```python
from build123d import *

# Parameters (mm, degrees)
SKETCH1_R           = 22.5
BOSS_EXTRUDE1_DEPTH = 20
SKETCH2_R           = 30
BOSS_EXTRUDE2_DEPTH = 40
SKETCH3_R           = 25
BOSS_EXTRUDE3_DEPTH = 30
SKETCH4_R           = 20
BOSS_EXTRUDE4_DEPTH = 25
SKETCH5_R           = 15
CUT_EXTRUDE1_DEPTH  = 116


with BuildPart() as part:
    # Sketch1 → Boss-Extrude1 (new body)
    with BuildSketch(Plane(origin=(0, 0, 0), x_dir=(0, 0, -1), z_dir=(1, 0, 0))):
        Circle(SKETCH1_R)
    extrude(amount=BOSS_EXTRUDE1_DEPTH)

    # Sketch2 → Boss-Extrude2 (add)
    with BuildSketch(Plane(origin=(20, 0, 0), x_dir=(0, 0, -1), z_dir=(1, 0, 0))):
        Circle(SKETCH2_R)
    extrude(amount=BOSS_EXTRUDE2_DEPTH)

    # Sketch3 → Boss-Extrude3 (add)
    with BuildSketch(Plane(origin=(60, 0, 0), x_dir=(0, 0, -1), z_dir=(1, 0, 0))):
        Circle(SKETCH3_R)
    extrude(amount=BOSS_EXTRUDE3_DEPTH)

    # Sketch4 → Boss-Extrude4 (add)
    with BuildSketch(Plane(origin=(90, 0, 0), x_dir=(0, 0, -1), z_dir=(1, 0, 0))):
        Circle(SKETCH4_R)
    extrude(amount=BOSS_EXTRUDE4_DEPTH)

    # Sketch5 → Cut-Extrude1 (cut, through all)
    with BuildSketch(Plane(origin=(115, 0, 0), x_dir=(0, 0, -1), z_dir=(1, 0, 0))):
        Circle(SKETCH5_R)
    extrude(amount=-CUT_EXTRUDE1_DEPTH, mode=Mode.SUBTRACT)


solid = part.part
```
Source: CAD feature listing. Evaluate the final solid. Frame: model axes, mm. A direction names the side the tool comes from. Round coordinates to 2 decimals unless told otherwise and drop trailing zeros. Order: outer loops, then holes, each group sorted by start corner. A loop starts at its lowest first (then second) coordinate and runs counter-clockwise, first axis right, second up. Notation, with made-up numbers: (-10, 71) -> (0, 71) arc R20 cw to (0, 105) -> close; hole circle Ø4 at (80.5, -15.75). An arc over 180 degrees is marked (long way). Use CSV: the item, a comma, the result in double quotes.
(1) Pull-direction query (Z, two-part tool) for faces 4 (the face through (9.86, -19.961, -10.382)), 5 (the face through (90, 17, 11)), 6 (the face through (58.305, 0.66, 14.985)); classes: +Z half, -Z half, draft (parallel to the pull), parting line (faces both ways), or undercut.
Report:
face 4,"parting line"
face 5,"draft"
face 6,"undercut"
(2) Section A-A on z = 0. Return the cut outline in (x, y), and give its area (3 significant figures).
Report:
outline,"(0, -22.5) -> (20, -22.5) -> (20, -30) -> (60, -30) -> (60, -25) -> (90, -25) -> (90, -20) -> (115, -20) -> (115, -15) -> (0, -15) -> close; (0, 15) -> (115, 15) -> (115, 20) -> (90, 20) -> (90, 25) -> (60, 25) -> (60, 30) -> (20, 30) -> (20, 22.5) -> (0, 22.5) -> close"
area,"2,350 mm^2"
(3) First-contact query: pin 1 Ø4 at (x, y) = (103, 14) entering from -Z; pin 2 Ø25 at (y, z) = (7, 12.5) entering from +X; pin 3 Ø2 at (x, z) = (30, 7) entering from -Y; pin 4 Ø12 at (x, z) = (94.5, -23) entering from +Y. Flat tips, straight axial feed; report the tip coordinate or a pass-through.
Report:
pin 1,"z = -16"
pin 2,"x = 115"
pin 3,"y = -29.39"
pin 4,"y = 16.21"
(4) Section C-C on x = 103. Return the cut outline in (y, z), and give its area (3 significant figures).
Report:
outline,"circle Ø40 at (0, 0); hole circle Ø30 at (0, 0)"
area,"550 mm^2"
(5) Section D-D on y = -17. Return the cut outline in (x, z), and give its area (3 significant figures).
Report:
outline,"(0, -14.74) -> (20, -14.74) -> (20, -24.72) -> (60, -24.72) -> (60, -18.33) -> (90, -18.33) -> (90, -10.54) -> (115, -10.54) -> (115, 10.54) -> (90, 10.54) -> (90, 18.33) -> (60, 18.33) -> (60, 24.72) -> (20, 24.72) -> (20, 14.74) -> (0, 14.74) -> close"
area,"4,190 mm^2"
(6) Access query for faces 1 (the face through (39.72, 1.32, 29.97)), 2 (the face through (60, 25, 7)), 3 (the face through (20, 22.4, -4.3)). Directions: +Z, -Z, +X, -X, +Y, -Y. A direction counts if a zero-diameter tool reaches every point of the face in a straight line with its end or side. Return the directions, or none.
Report:
face 1,"+X, -X"
face 2,"+X"
face 3,"-X"
(7) Ray query, L1, parallel to Y at x = 80.5, z = 0; L2, parallel to Y at x = 36, z = 0; L3, parallel to Z at x = 8.5, y = 4. Return the intervals inside material, ascending.
Report:
L1,"-25 to -15, 15 to 25"
L2,"-30 to -15, 15 to 30"
L3,"-22.14 to -14.46, 14.46 to 22.14"
